Could you check a few things on this model? Use its own coordinates, in mm. Round coordinates to 2 decimals unless told otherwise and drop trailing zeros. Write each loop counter-clockwise with the first axis right and the second up, starting at its lowest first coordinate (ties: lowest second). Pieces come first, ordered by that corner, then holes. Notation, with made-up numbers: (-21, 1) -> (38, 1) arc R8 ccw to (38, 12) -> close; hole circle Ø9 at (-34, 50). An arc over 180 degrees is marked (long way). Return JSON: item names as keys, results as strings.
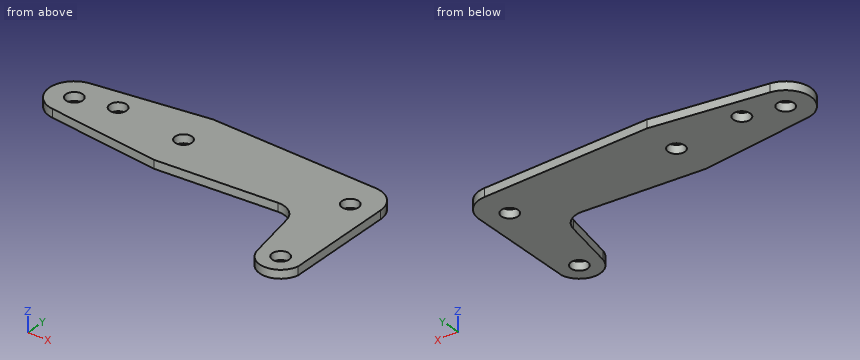
from build123d import *

# Parameters (mm, degrees)
BOSS_EXTRUDE1_DEPTH = 3.175
SKETCH2_R           = 3.175
CUT_EXTRUDE1_DEPTH  = 87.033766175


with BuildPart() as part:
    # Sketch1 → Boss-Extrude1 (new body)
    with BuildSketch(Plane.XY):
        with BuildLine():
            Line((-42.82323198, 9.447015826), (-0.046249169, 14.954781853))
            Line((-0.046249169, 14.954781853), (63.914748375, 12.26924))
            ThreePointArc((63.914748375, 12.26924), (70.390184722, 9.345032033), (73.04017255, 2.752624837))
            Line((73.04017255, 2.752624837), (73.04017255, -38.893945713))
            ThreePointArc((73.04017255, -38.893945713), (65.231134486, -45.352634886), (57.422096421, -38.893945713))
            Line((57.422096421, -38.893945713), (53.624835968, -19.012795079))
            ThreePointArc((53.624835968, -19.012795079), (50.720085476, -14.247018679), (45.398312666, -12.56507508))
            Line((45.398312666, -12.56507508), (-0.046249169, -14.954781853))
            Line((-0.046249169, -14.954781853), (-42.82323198, -9.447015826))
            ThreePointArc((-42.82323198, -9.447015826), (-51.131878011, 0), (-42.82323198, 9.447015826))
        make_face()
    extrude(amount=BOSS_EXTRUDE1_DEPTH)

    # Sketch2 → Cut-Extrude1 (cut, through all)
    with BuildSketch(Plane.XY.offset(3.175)):
        with Locations((-41.606878011, 0)):
            Circle(SKETCH2_R)
        with Locations((-27.306678011, 3.175)):
            Circle(SKETCH2_R)
        Circle(SKETCH2_R)
        with Locations((63.5, 0.037204921)):
            Circle(SKETCH2_R)
        with Locations((65.231134486, -37.402434886)):
            Circle(SKETCH2_R)
    extrude(amount=-CUT_EXTRUDE1_DEPTH, mode=Mode.SUBTRACT)


solid = part.part
1) If I drill on probe 1 along Y at (x, z) = (0, 0.95) (3 decimals); probe 2 along Y at (x, z) = (62.5, 0.8); probe 3 along Y at (x, z) = (65, 0.9), over which ranges is the centre line in solid material (lowest first)? Write a range as [from, to].
Return value:
{"probe 1": "[-14.952, -3.175], [3.175, 14.953]", "probe 2": "[-44.87, -39.02], [-35.78, -2.98], [3.05, 12.33]", "probe 3": "[-45.35, -40.57], [-34.24, -2.76], [2.84, 12.16]"}
2) I want a section at C-C, the plane x = 34. Please give me the cut outline in (y, z) (3 decimals), and give its area (3 significant figures).
Return value:
{"outline": "(-13.164, 0) -> (13.525, 0) -> (13.525, 3.175) -> (-13.164, 3.175) -> close", "area": "84.7 mm²"}
3) I want a section at B-B, the plane x = -9.5. Please give me the cut outline in (y, z) (3 decimals), and give its area (3 significant figures).
Return value:
{"outline": "(-13.738, 0) -> (13.738, 0) -> (13.738, 3.175) -> (-13.738, 3.175) -> close", "area": "87.2 mm²"}
4) I want a section at A-A, the plane z = 2.5. Please give me the cut outline in (x, y) (3 decimals).
Return value:
{"outline": "(-42.823, -9.447) -> (-0.046, -14.955) -> (45.398, -12.565) arc R7.95 cw to (53.625, -19.013) -> (57.422, -38.894) arc R7.95 ccw to (73.04, -38.894) -> (73.04, 2.753) arc R9.525 ccw to (63.915, 12.269) -> (-0.046, 14.955) -> (-42.823, 9.447) arc R9.525 ccw to start; hole circle Ø6.35 at (-41.607, 0); hole circle Ø6.35 at (-27.307, 3.175); hole circle Ø6.35 at (0, 0); hole circle Ø6.35 at (63.5, 0.037); hole circle Ø6.35 at (65.231, -37.402)"}
5) Will these pins go through, and if not, where does the flat tip stop? pin 1 Ø1 at (x, z) = (5, 1) entering from +Y; pin 2 Ø1.5 at (x, z) = (49, 2) entering from -Y.
Return value:
{"pin 1": "y = 14.76", "pin 2": "y = -13.6"}
